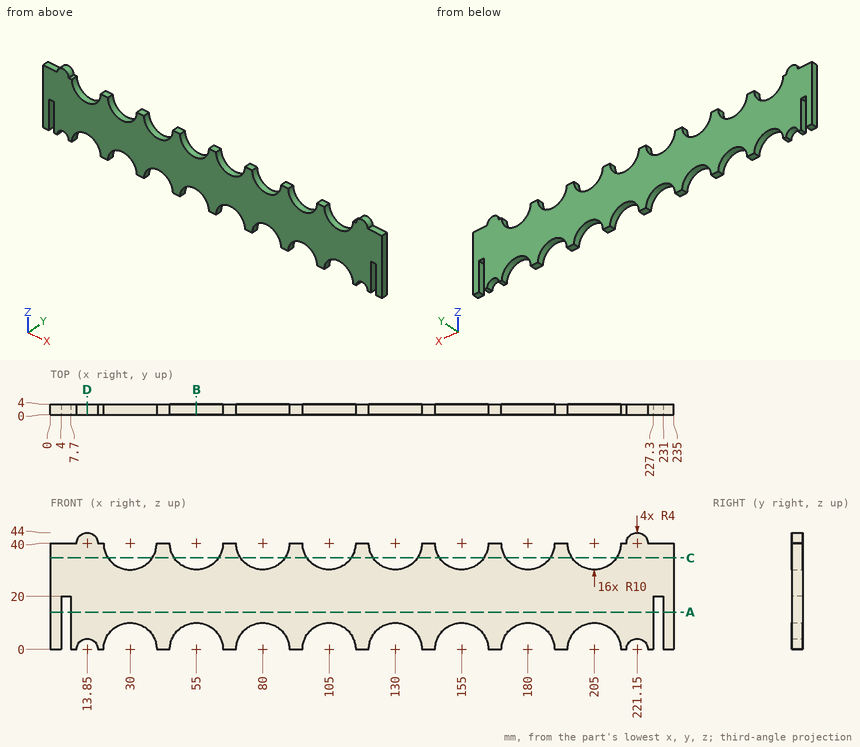
Study the drawing (mm; zero at the part's minimum x, y, z) and answer. Round coordinates to 2 decimals unless told otherwise and drop trailing zeros. Loops run counter-clockwise (first coordinate to the right, second up) from the corner with the lowest first, then second, coordinate; pieces in that order, holes last. Notation, with made-up numbers: M 59.25,-22 L 102.25,-22 A31 cw 102.25,17 Z; hole C 21.5,30.5 d10. An arc over 180 degrees is marked long. One line per question, with ' | ' between items.
Q1. Find section B-B, the plane x = 55. Give the vertices of the cut face in (y, z), then the cut area to 3 significant figures.
Conclusion:
outline: M 0,10 L 4,10 L 4,30 L 0,30 Z | area: 80.0 mm2
Q2. Find section D-D, the plane x = 13.85. Give the vertices of the cut face in (y, z).
Conclusion:
outline: M 0,4 L 4,4 L 4,44 L 0,44 Z
Q3. Consider line 1 along X through (y, z) = (1.2, 14); line 2 along Z through (x, y) = (167, 0.6); line 3 along Z through (x, y) = (129.5, 3.15). Determine where each line is inside the solid, lowest interval first. Write a range as from..to.
Conclusion:
line 1: x = 0..4, 7.7..227.3, 231..235 | line 2: z = 0..40 | line 3: z = 9.99..30.01
Q4. Each of these flat-tipped pins is pushed along its axis until it touches: pin 1 Ø2 at (x, y) = (228, 3) entering from +Z; pin 2 Ø1.1 at (x, y) = (5.5, 2.5) entering from -Z. Where does it stop, or does it pass through?
Conclusion:
pin 1: stops at z = 40 | pin 2: stops at z = 20
Q5. Find section A-A, the plane z = 14. Give the vertices of the cut face in (x, y).
Conclusion:
outline: M 0,0 L 4,0 L 4,4 L 0,4 Z; M 7.7,0 L 227.3,0 L 227.3,4 L 7.7,4 Z; M 231,0 L 235,0 L 235,4 L 231,4 Z
Q6. Find section C-C, the plane z = 34.5. State how many separate pieces and enclosed holes the cut face has, then the cut area to 3 significant figures.
Conclusion:
separate pieces: 9 | enclosed holes: 0 | area: 405 mm2
